from build123d import *

# Parameters (mm, degrees)
SKETCH1_W            = 17.6
SKETCH1_H            = 15
BOSS_EXTRUDE1_DEPTH  = 1.5
SKETCH2_W            = 14.8
SKETCH2_H            = 10
CUT_EXTRUDE1_DEPTH   = 1.4
SKETCH3_R            = 0.7
BOSS_EXTRUDE2_DEPTH  = 1.5
SKETCH4_R            = 0.7
BOSS_EXTRUDE3_DEPTH  = 0.5
FILLET2_R            = 0.5
FILLET2_OF_MIRROR1_R = 0.5
FILLET1_R            = 0.5


with BuildPart() as part:
    # Sketch1 → Boss-Extrude1 (new, symmetric)
    with BuildSketch(Plane(origin=(0, 0, 0), x_dir=(1, 0, 0), z_dir=(0, 1, 0))):
        Rectangle(SKETCH1_W, SKETCH1_H)
    extrude(amount=BOSS_EXTRUDE1_DEPTH, both=True)

    # Sketch2 → Cut-Extrude1 (cut)
    with BuildSketch(Plane.XZ.offset(1.5)):
        Rectangle(SKETCH2_W, SKETCH2_H)
    extrude(amount=-CUT_EXTRUDE1_DEPTH, mode=Mode.SUBTRACT)

    # Sketch3 → Boss-Extrude2 (add)
    with BuildSketch(Plane.ZY.offset(8.8)):
        with Locations(Location((-6.1, 0, 0), (0, 0, 180))):
            Circle(SKETCH3_R)
    boss_extrude2 = extrude(amount=BOSS_EXTRUDE2_DEPTH)

    # Sketch4 → Boss-Extrude3 (add)
    with BuildSketch(Plane.ZY.offset(8.8)):
        with Locations(Location((3.9, 0, 0), (0, 0, 180))):
            Circle(SKETCH4_R)
    boss_extrude3 = extrude(amount=BOSS_EXTRUDE3_DEPTH)

    # Fillet2
    fillet2_edges = [part.edges().sort_by_distance(p)[0] for p in [
        (-9.3, 0, 4.6),
    ]]
    fillet(fillet2_edges, radius=FILLET2_R - 0.0001)  # a hair under: the kernel refuses the full size

    # Mirror1: Boss-Extrude2, Boss-Extrude3 across plane
    add(boss_extrude2.mirror(Plane(origin=(0, 0, 0), x_dir=(0, 0, 1), z_dir=(1, 0, 0))))
    add(boss_extrude3.mirror(Plane(origin=(0, 0, 0), x_dir=(0, 0, 1), z_dir=(1, 0, 0))))

    # Fillet2 of Mirror1
    fillet2_of_mirror1_edges = [part.edges().sort_by_distance(p)[0] for p in [
        (9.3, 0, 4.6),
    ]]
    fillet(fillet2_of_mirror1_edges, radius=FILLET2_OF_MIRROR1_R - 0.0001)  # a hair under: the kernel refuses the full size

    # Fillet1
    fillet1_edges = [part.edges().sort_by_distance(p)[0] for p in [
        (0, 1.5, 7.5),
        (0, -1.5, 7.5),
        (0, -1.5, -7.5),
        (0, 1.5, -7.5),
    ]]
    fillet(fillet1_edges, radius=FILLET1_R)


solid = part.part
Geometry check sheet. Reference: the model listing, model coordinates, mm. A direction names the side the tool comes from. Round coordinates to 2 decimals unless told otherwise and drop trailing zeros. Order: outer loops, then holes, each group sorted by start corner. A loop starts at its lowest first (then second) coordinate and runs counter-clockwise, first axis right, second up. Notation, with made-up numbers: M 19,5.25 L 52,5.25 A25 ccw 52,30.25 Z; hole C 58.25,-11 d3. An arc over 180 degrees is marked long. Write each question's results on one line, items separated by ' | '. Start each with the question number.
1. Cross-section at A-A on z = -6.1. Record the boundary of the cut face in (x, y), plus the area to 3 significant figures.
2. Material ranges on L1, parallel to Z at x = -1.25, y = -0.95; L2, parallel to X at y = -0.75, z = -4.25; L3, parallel to Z at x = -3.5, y = -1.3, recorded low to high. Write a range as from..to.
3. Set-up check for faces 4 (the face through (10.3, 0, -6)), 5 (the face through (9.54, -0.21, -6.768)), 6 (the face through (-9.54, -0.21, -6.768)), 7 (the face through (7.4, -1, 0)): record each of +Z, -Z, +X, -X, +Y, -Y from which the full face is reachable in a straight line by a thin tool's end or side.
4. Cross-section at C-C on z = -4.25. Record the boundary of the cut face in (x, y).
5. Draft check along Z on faces 1 (the face through (0, -1.5, 6)), 2 (the face through (8.8, 0, 0)), 3 (the face through (0, 0, -7.5)). Enter one of: pulls with the +Z half, pulls with the -Z half, needs draft (parallel to the pull), parting line crosses it, or undercut.
6. Cross-section at D-D on z = 6. Record the boundary of the cut face in (x, y), plus the area to 3 significant figures.
7. Cross-section at B-B on x = -1.25. Record the boundary of the cut face in (y, z), plus the area to 3 significant figures.
8. Go/stop test with flat-tipped pins: P1, Ø0.9, axis at y = 0, z = 1, coming from the -X side; P2, Ø1.1, axis at y = -0.5, z = 2, coming from the +X side. Record where each tip stops, or that it passes through.
Resolved:
1) outline: M -10.3,-0.7 L -8.8,-0.7 L -8.8,-1.5 L 8.8,-1.5 L 8.8,-0.7 L 10.3,-0.7 L 10.3,0.7 L 8.8,0.7 L 8.8,1.5 L -8.8,1.5 L -8.8,0.7 L -10.3,0.7 Z | area: 57.0 mm2
2) L1: -7.5..-5, 5..7.5 | L2: -8.8..-7.4, 7.4..8.8 | L3: -7.4..-5, 5..7.4
3) face 4: +Z, -Z, +X, +Y, -Y | face 5: +X | face 6: -X | face 7: -Y
4) outline: M -8.8,-1.5 L -7.4,-1.5 L -7.4,-0.1 L 7.4,-0.1 L 7.4,-1.5 L 8.8,-1.5 L 8.8,1.5 L -8.8,1.5 Z
5) face 1: needs draft | face 2: undercut | face 3: pulls with the -Z half
6) outline: M -8.8,-1.5 L 8.8,-1.5 L 8.8,1.5 L -8.8,1.5 Z | area: 52.8 mm2
7) outline: M -1.5,-7 A0.5 ccw -1,-7.5 L 1,-7.5 A0.5 ccw 1.5,-7 L 1.5,7 A0.5 ccw 1,7.5 L -1,7.5 A0.5 ccw -1.5,7 L -1.5,5 L -0.1,5 L -0.1,-5 L -1.5,-5 Z | area: 30.8 mm2
8) P1: x = -8.8 | P2: x = 8.8
